Check sheet for the drawn part. Datum: minimum x, y, z corner. Units: mm. A direction names the side the tool comes from. Coordinates: 2 decimals unless noted, no trailing zeros. Write each loop counter-clockwise with the first axis right and the second up, starting at its lowest first coordinate (ties: lowest second). Pieces come first, ordered by that corner, then holes. Notation, with made-up numbers: M 15,38.5 L 20,38.5 A19 cw 20,71.5 Z; hole C 37.25,82.25 d2. An arc over 180 degrees is marked long. Answer as CSV lines item,"result". Start each with the question number.
Q1. Thickness scan on line 1 along Z through (x, y) = (21, 3); line 2 along Y through (x, z) = (29.5, 5) (1 decimal); line 3 along X through (y, z) = (25.5, 29.5). Record the ranges inside material, lowest first. Write a range as from..to.
Q2. Sectioned sample at B-B, the plane z = 8. Record the cut outline in (x, y), then the cut area to 3 significant figures.
Q3. Sectioned sample at A-A, the plane z = 32. Record the cut outline in (x, y) (1 decimal).
Q4. Depth check by flat-ended pin: pin 1 Ø8 at (y, z) = (6.5, 34) entering from -X; pin 2 Ø8 at (y, z) = (13, 17) entering from -X; pin 3 Ø1 at (x, z) = (7.5, 15.5) entering from -Y. Enter the tip coordinate at first touch or a pass-through.
Q5. Access from +Z, -Z, +X, -X, +Y, -Y to the whole of each face (thin tool, end or side, straight path). Record for the marked faces 1, 2 and 3.
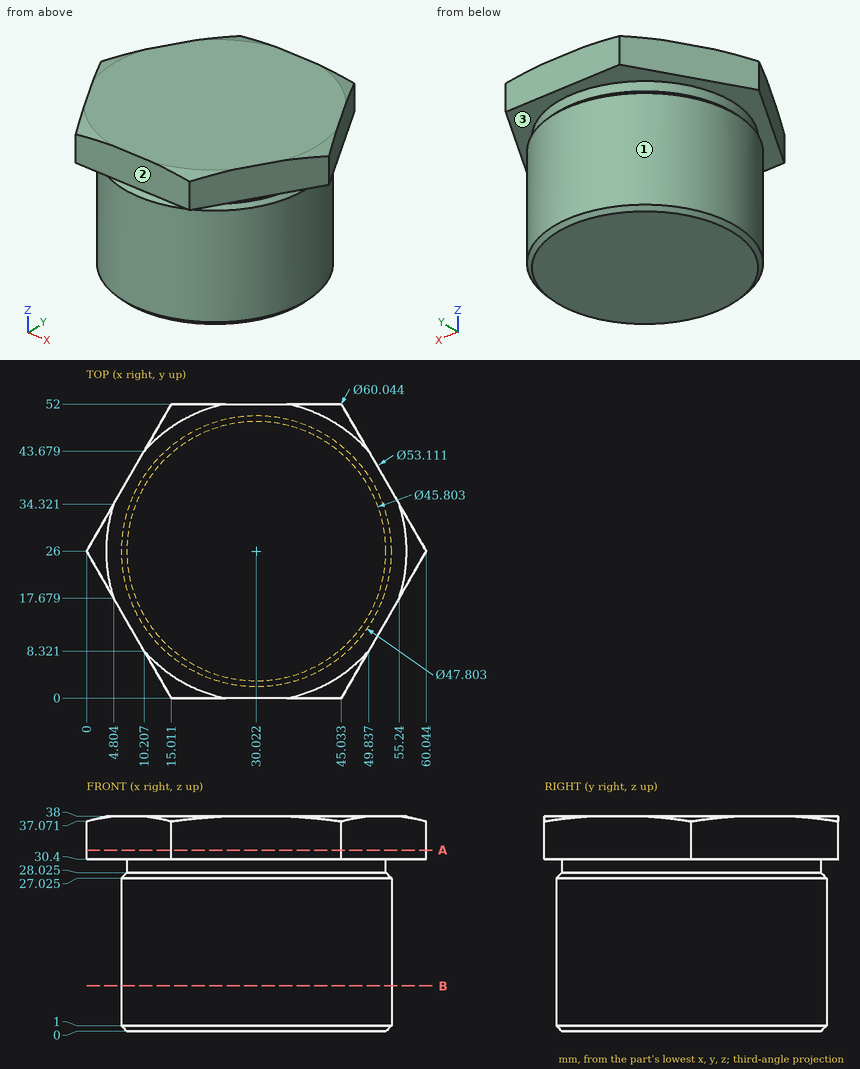
Output:
1,line 1,"z = 30.4..38"
1,line 2,"y = 2.1..49.9"
1,line 3,"x = 7.13..52.92"
2,outline,"C 30.02,26 d47.8"
2,area,"1,790 mm^2"
3,outline,"M 0,26 L 15,0 L 45,0 L 60,26 L 45,52 L 15,52 Z"
4,pin 1,"stops at x = 8.95"
4,pin 2,"stops at x = 7.88"
4,pin 3,"stops at y = 16.71"
5,face 1,"-Z"
5,face 2,"+Z, -Z, +X, -X, -Y"
5,face 3,"none"
